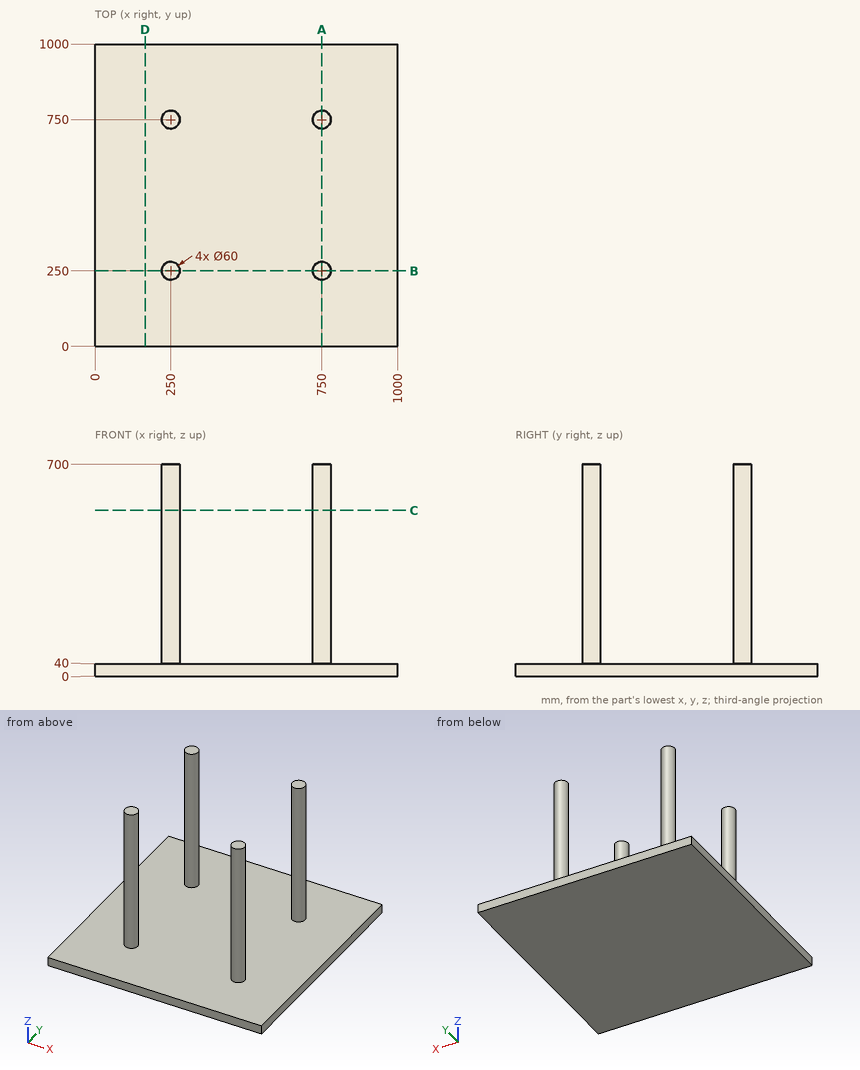
Print and shaded views of the part. All mm, measured from the part's lowest x, y and z. Give positions to 0.01 mm unless a question says otherwise; leave off trailing zeros. Loops run counter-clockwise (first coordinate to the right, second up) from the corner with the lowest first, then second, coordinate; pieces in that order, holes last. Notation, with made-up numbers: (-39, 12) -> (-8, 12) arc R28 ccw to (-8, 42) -> close; hole circle Ø4 at (32.25, 66). An arc over 180 degrees is marked (long way). Use a Markdown table: item, result.
1. Flat gauge pins, fed straight in: pin 1 (12 mm diameter, centred on x = 474.5, y = 117, fed in from -Z); pin 2 (8 mm diameter, centred on x = 402.5, y = 625.5, fed in from +Z). Where does each tip first touch, or does it go through?
Check result:
| item | result |
|---|---|
| pin 1 | stops at z = 0 |
| pin 2 | stops at z = 40 |
2. Slice it at A-A (x = 750). List the corners of the cut face in (y, z).
Check result:
| item | result |
|---|---|
| outline | (0, 0) -> (1000, 0) -> (1000, 40) -> (780, 40) -> (780, 700) -> (720, 700) -> (720, 40) -> (280, 40) -> (280, 700) -> (220, 700) -> (220, 40) -> (0, 40) -> close |
3. Wall check: L1, parallel to Z at x = 109.5, y = 559.5; L2, parallel to X at y = 268.5, z = 479.5; L3, parallel to Y at x = 740, z = 640. Give the ranges that are in metal, low to high. Write a range as [from, to].
Check result:
| item | result |
|---|---|
| L1 | z = [0, 40] |
| L2 | x = [226.38, 273.62], [726.38, 773.62] |
| L3 | y = [221.72, 278.28], [721.72, 778.28] |
4. Slice it at D-D (x = 165). List the corners of the cut face in (y, z).
Check result:
| item | result |
|---|---|
| outline | (0, 0) -> (1000, 0) -> (1000, 40) -> (0, 40) -> close |
5. Slice it at C-C (z = 548). List the corners of the cut face in (x, y).
Check result:
| item | result |
|---|---|
| outline | circle Ø60 at (250, 250); circle Ø60 at (250, 750); circle Ø60 at (750, 250); circle Ø60 at (750, 750) |
